from build123d import *

# Parameters (mm, degrees)
SKETCH1_W           = 20
SKETCH1_H           = 20
SKETCH1_W_2         = 17
SKETCH1_H_2         = 17
BOSS_EXTRUDE1_DEPTH = 220
SKETCH2_R           = 2.125
CUT_EXTRUDE1_DEPTH  = 222.133443875


with BuildPart() as part:
    # Sketch1 → Boss-Extrude1 (new body)
    with BuildSketch(Plane.XY):
        Rectangle(SKETCH1_W, SKETCH1_H)
        Rectangle(SKETCH1_W_2, SKETCH1_H_2, mode=Mode.SUBTRACT)
    extrude(amount=-BOSS_EXTRUDE1_DEPTH)

    # Sketch2 → Cut-Extrude1 (cut, through all)
    with BuildSketch(Plane(origin=(0, 10, 0), x_dir=(1, 0, 0), z_dir=(0, 1, 0))):
        with Locations(Location((0, 10, 0), (0, 0, 270))):
            Circle(SKETCH2_R)
        with Locations(Location((0, 110, 0), (0, 0, 270))):
            Circle(SKETCH2_R)
        with Locations(Location((0, 210, 0), (0, 0, 270))):
            Circle(SKETCH2_R)
        with Locations(Location((0, 25, 0), (0, 0, 270))):
            Circle(SKETCH2_R)
        with Locations(Location((0, 195, 0), (0, 0, 90))):
            Circle(SKETCH2_R)
    extrude(amount=-CUT_EXTRUDE1_DEPTH, mode=Mode.SUBTRACT)


solid = part.part
The model under review builds one solid part; all positions refer to its coordinate system, in mm. A direction names the side the tool comes from. Round coordinates to 2 decimals unless told otherwise and drop trailing zeros. Write each loop counter-clockwise with the first axis right and the second up, starting at its lowest first coordinate (ties: lowest second). Pieces come first, ordered by that corner, then holes. Notation, with made-up numbers: M -12,73 L 8,73 A23 ccw 8,94 Z; hole C -4.75,89.25 d4. An arc over 180 degrees is marked long. Answer as CSV lines item,"result". Start each with the question number.
Q1. Clearance check with flat-ended pins moving along their axes: P1, Ø3.5, axis at x = 0, z = -10, coming from the -Y side; P2, Ø5.5, axis at x = 0, z = -10, coming from the -Y side. State where each tip first meets the part, or that it passes through.
Q2. The part is to be moulded in two halves that separate along Z. For faces 3 (the face through (0.093, 9.26, -212.123)), 4 (the face through (-9, 0, -220)), 5 (the face through (-8.5, 0, -108)), say which applies: +Z half, -Z half, draft (parallel to the pull), parting line (faces both ways), or undercut.
Q3. Consider section A-A, the plane x = -6.25. Give the boundary of the cut face in (y, z).
Q4. Tool access review of faces 1 (the face through (-2, 8.5, -108)), 2 (the face through (2, 10, -108)): name each direction out of +Z, -Z, +X, -X, +Y, -Y from which nothing blocks a thin tool from reaching the whole face with its end or side.
Q5. Consider section C-C, the plane z = -110. Give the boundary of the cut face in (x, y) (3 decimals), then the cut area to 4 significant figures.
Q6. Consider section D-D, the plane z = -141. Give the boundary of the cut face in (x, y).
Q7. Wall thickness on line 1 along X through (y, z) = (3.75, -70.5); line 2 along X through (y, z) = (9.1, -110) (3 decimals): over which ranges is each line inside the solid? List them lowest first.
Result set:
1,P1,"passes through"
1,P2,"stops at y = -10"
2,face 3,"undercut"
2,face 4,"-Z half"
2,face 5,"draft"
3,outline,"M -10,-220 L -8.5,-220 L -8.5,0 L -10,0 Z; M 8.5,-220 L 10,-220 L 10,0 L 8.5,0 Z"
4,face 1,"+Z, -Z"
4,face 2,"+Z, -Z, +X, -X, +Y"
5,outline,"M -10,-10 L -2.125,-10 L -2.125,-8.5 L -8.5,-8.5 L -8.5,8.5 L -2.125,8.5 L -2.125,10 L -10,10 Z; M 2.125,-10 L 10,-10 L 10,10 L 2.125,10 L 2.125,8.5 L 8.5,8.5 L 8.5,-8.5 L 2.125,-8.5 Z"
5,area,"98.25 mm²"
6,outline,"M -10,-10 L 10,-10 L 10,10 L -10,10 Z; hole M -8.5,-8.5 L 8.5,-8.5 L 8.5,8.5 L -8.5,8.5 Z"
7,line 1,"x = -10 to -8.5, 8.5 to 10"
7,line 2,"x = -10 to -2.125, 2.125 to 10"
